The model under review builds one solid part; all positions refer to its coordinate system, in mm. Coordinates: 2 decimals unless noted, no trailing zeros. Loops run counter-clockwise (first coordinate to the right, second up) from the corner with the lowest first, then second, coordinate; pieces in that order, holes last. Notation, with made-up numbers: (-4.5, 76) - (54.5, 76) arc R14 ccw to (54.5, 102) - close; hole circle Ø1 at (1, 18). An arc over 180 degrees is marked (long way). Answer in a Markdown table with one row per item. Add a question column.
(1) We need section D-D on y = 1.5. Write out the cut boundary in (x, z) (3 decimals), plus the area to 3 significant figures.
(2) For P1, Ø1, axis at y = -3.5, z = 34, coming from the -X side; P2, Ø20.5, axis at x = 1, z = 34, coming from the +Y side; P3, Ø8, axis at y = 5.5, z = 20, coming from the +X side, all flat-tipped, find the tip position at first contact; note any pin that passes through.
(3) We need section C-C on z = 38. Write out the cut boundary in (x, y), plus the area to 3 significant figures.
(4) For line 1 along Y through (x, z) = (-11, 50.5); line 2 along Z through (x, y) = (0, -2.5) (3 decimals); line 3 along X through (y, z) = (-12, -6), list the stretches that pass through material, from the lowest coordinate up.
(5) We need section B-B on z = 0. Write out the cut boundary in (x, y) (3 decimals).
(6) Mouldability with a two-part tool opening along X and no side actions: class faces 1 (the flat face through (13.849, 0, 35)), 2 (the cylindrical face through (-7.559, -0.221, -5.796)), 3 (the flat face through (1, 6.35, 35)), 4 (the flat face through (-11.551, 0, 36)) as +X half, -X half, draft (parallel to the pull), parting line (faces both ways), or undercut.
(7) We need section A-A on x = 0. Write out the cut boundary in (y, z) (3 decimals).
from build123d import *

# Parameters (mm, degrees)
F3_DEPTH = 59.944
F4_R     = 9.525
F5_DEPTH = 38.1


with BuildPart() as f1:
    # F0 (on Right) → F1 (revolve)
    with BuildSketch(Plane.YZ):
        with BuildLine():
            Line((0, 0), (0, -18.415))
            ThreePointArc((0, -18.415), (18.415, 0), (0, 18.415))
            Line((0, 18.415), (0, 0))
        make_face()
    revolve(axis=Axis((0, 0, -9.2075), (0, 0, -1)))

    # F2 (on Top) → F3 (join)
    with BuildSketch(Plane.XY):
        Polygon((13.84911329, 6.35), (-11.55088671, 6.35), (-11.55088671, -6.35), (0, -6.35), (13.84911329, -6.35), align=None)
    extrude(amount=F3_DEPTH)

    # F4 (on Front) → F5 (cut, symmetric)
    with BuildSketch(Plane.XZ):
        Circle(F4_R)
    extrude(amount=F5_DEPTH, both=True, mode=Mode.SUBTRACT)


solid = f1.part
Outcome:
| question | item | result |
|---|---|---|
| 1 | outline | (-11.551, 14.263) arc R18.354 ccw (long way) to (13.849, 12.044) - (13.849, 59.944) - (-11.551, 59.944) - close; hole circle Ø19.05 at (0, 0) |
| 1 | area | 1,870 mm² |
| 2 | P1 | x = -11.55 |
| 2 | P2 | y = 6.35 |
| 2 | P3 | x = 13.85 |
| 3 | outline | (-11.55, -6.35) - (13.85, -6.35) - (13.85, 6.35) - (-11.55, 6.35) - close |
| 3 | area | 323 mm² |
| 4 | line 1 | -6.35 to 6.35 |
| 4 | line 2 | -18.245 to -9.525, 9.525 to 59.944 |
| 4 | line 3 | -12.61 to -7.4, 7.4 to 12.61 |
| 5 | outline | (-9.525, -15.76) - (-9.525, 15.76) arc R18.415 ccw to start; (9.525, -15.76) arc R18.415 ccw to (9.525, 15.76) - close |
| 6 | face 1 | +X half |
| 6 | face 2 | undercut |
| 6 | face 3 | draft |
| 6 | face 4 | -X half |
| 7 | outline | (-15.76, -9.525) arc R18.415 ccw to (15.76, -9.525) - close; (-15.76, 9.525) - (15.76, 9.525) arc R18.415 ccw to (6.35, 17.286) - (6.35, 59.944) - (-6.35, 59.944) - (-6.35, 17.286) arc R18.415 ccw to start |
